```python
from build123d import *

# Parameters (mm, degrees)
F0_R            = 16.8606013276
F0_R_2          = 1.7272
F0_R_3          = 4.7625
F1_DEPTH        = 3.175
F3_DEPTH        = 3.175
F3_COPIES_COUNT = 34


# Not quite as in the source:
# - a pattern or mirror of a feature is missing from the dataset's text; its kind, count and spacing are read off the source's solid
# - a feature names something its author has since deleted; it is built from what else it names


with BuildPart() as f1:
    # F0 (on Top) → F1 (new body)
    with BuildSketch(Plane.XY):
        Circle(F0_R)
        with Locations((0, -10.31875)):
            Circle(F0_R_2, mode=Mode.SUBTRACT)
        Circle(F0_R_3, mode=Mode.SUBTRACT)
        with Locations((0, 10.31875)):
            Circle(F0_R_2, mode=Mode.SUBTRACT)
    extrude(amount=F1_DEPTH)

    # F2 (on face) → F3 (cut, through all)
    with BuildSketch(Plane.XY.offset(3.175)):
        with BuildLine():
            Line((0.2750051008, 14.882965874), (1.0776094804, 16.8261295293))
            ThreePointArc((1.0776094804, 16.8261295293), (0, 16.8606013276), (-1.0776094804, 16.8261295293))
            Line((-1.0776094804, 16.8261295293), (-0.2750051008, 14.882965874))
            ThreePointArc((-0.2750051008, 14.882965874), (0, 14.6990139664), (0.2750051008, 14.882965874))
        make_face()
    f3 = extrude(amount=-F3_DEPTH, mode=Mode.SUBTRACT)

    # F3_copies: F3 ×34 about axis
    f3_copies_axis = Axis((0, 0, 0), (0, 0, 1))
    for i in range(1, F3_COPIES_COUNT):
        add(f3.rotate(f3_copies_axis, i * 360 / F3_COPIES_COUNT), mode=Mode.SUBTRACT)


solid = f1.part
```
Build history of the part. All positions in model axes, mm. A direction names the side the tool comes from. Round coordinates to 2 decimals unless told otherwise and drop trailing zeros. Write each loop counter-clockwise with the first axis right and the second up, starting at its lowest first coordinate (ties: lowest second). Pieces come first, ordered by that corner, then holes. Notation, with made-up numbers: (39.5, -38) - (46.5, -38) arc R9 cw to (46.5, -21) - close; hole circle Ø1 at (59.5, 57.25). An arc over 180 degrees is marked (long way). Write each question's results on one line, items separated by ' | '. Start each with the question number.
Item 1: Which spindle directions (+Z, -Z, +X, -X, +Y, -Y) get a long thin tool onto all of the face, cutting with end or side? Do faces 1 (the face through (-15.863, 0.785, 1.61)), 2 (the face through (-3.57, -15.45, 1.61)), 3 (the face through (13.9, 7.68, 1.61)), 4 (the face through (3.57, 15.45, 1.61)), 5 (the face through (7.77, -13.82, 1.61)). Say none if no direction does.
Item 2: Saw through at D-D (x = -6.5). Write the cut outline in (y, z) (3 decimals), and give its area (3 significant figures).
Item 3: Saw through at B-B (z = 0.5). State how many separate pieces and enclosed holes the cut face has, and give its area (3 significant figures).
Item 4: Wall check: L1, parallel to Y at x = 0, z = 1.5; L2, parallel to X at y = 14.5, z = 2.2; L3, parallel to Y at x = 15, z = 2.2. Give the ranges that are in metal, low to high. Write a range as [from, to].
Item 5: Saw through at A-A (y = 0). Write the cut outline in (x, z) (1 decimal), and give its area (3 significant figures).
Item 6: Drop flat-ended pins along their axis: P1, Ø2, axis at x = 0, y = -10.32, coming from the -Z side (1 decimal); P2, Ø6, axis at x = 3.5, y = 6, coming from the -Z side. Give the stop position or say it passes through.
Item 7: Saw through at C-C (x = 11). Write the cut outline in (y, z) (3 decimals).
Results are:
1) face 1: +Z, -Z, -X | face 2: +Z, -Z, -Y | face 3: +Z, -Z, +X | face 4: +Z, -Z, +Y | face 5: +Z, -Z
2) outline: (-14.689, 0) - (14.689, 0) - (14.689, 3.175) - (-14.689, 3.175) - close | area: 93.3 mm²
3) separate pieces: 1 | enclosed holes: 3 | area: 710 mm²
4) L1: y = [-14.7, -12.05], [-8.59, -4.76], [4.76, 8.59], [12.05, 14.7] | L2: x = [-7.88, -6.32], [-5.11, -2.93], [-2.58, 2.58], [2.93, 5.11], [6.32, 7.88] | L3: y = [-6.5, -4.94], [-3.74, -1.76], [-1.05, 1.05], [1.76, 3.74], [4.94, 6.5]
5) outline: (-16.9, 0) - (-4.8, 0) - (-4.8, 3.2) - (-16.9, 3.2) - close; (4.8, 0) - (16.9, 0) - (16.9, 3.2) - (4.8, 3.2) - close | area: 76.8 mm²
6) P1: passes through | P2: stops at z = 0
7) outline: (-11.176, 0) - (11.176, 0) - (11.176, 3.175) - (-11.176, 3.175) - close
